from build123d import *

# Parameters (mm, degrees)
EXTRUDE_1_DEPTH      = 5
EXTRUDE_1_DEPTH_BACK = 2
SKETCH_2_W           = 30
SKETCH_2_H           = 5
EXTRUDE_2_DEPTH      = 25
SKETCH_3_W           = 60
SKETCH_3_H           = 10
EXTRUDE_3_DEPTH      = 25


with BuildPart() as part:
    # 草圖1 → 填料-伸長1 (new, two sides: drawn at the far end of the back side and taken through both)
    with BuildSketch(Plane(origin=(0, 0, 0), x_dir=(1, 0, 0), z_dir=(0, 1, 0)).offset(-EXTRUDE_1_DEPTH_BACK)):
        Polygon((-60, 65), (-60, 40), (-30, 40), (-30, 65), (30, 65), (30, 40), (60, 40), (60, 65), (100, 65), (100, -65), (60, -65), (60, -40), (30, -40), (30, -65), (-30, -65), (-30, -40), (-60, -40), (-60, -65), (-100, -65), (-100, 65), align=None)
    extrude(amount=EXTRUDE_1_DEPTH + EXTRUDE_1_DEPTH_BACK)

    # 草圖2 → 填料-伸長2 (add)
    with BuildSketch(Plane(origin=(0, 5, 0), x_dir=(1, 0, 0), z_dir=(0, 1, 0))):
        with Locations((-45, 37.5)):
            Rectangle(SKETCH_2_W, SKETCH_2_H)
        with Locations((-45, -37.5)):
            Rectangle(SKETCH_2_W, SKETCH_2_H)
        with Locations((45, -37.5)):
            Rectangle(SKETCH_2_W, SKETCH_2_H)
        with Locations((45, 37.5)):
            Rectangle(SKETCH_2_W, SKETCH_2_H)
    extrude(amount=EXTRUDE_2_DEPTH)

    # 草圖3 → 填料-伸長3 (add)
    with BuildSketch(Plane(origin=(0, 5, 0), x_dir=(1, 0, 0), z_dir=(0, 1, 0))):
        Polygon((70, -65), (100, -65), (100, 65), (70, 65), (70, 55), (90, 55), (90, -55), (70, -55), align=None)
        with Locations((0, 60)):
            Rectangle(SKETCH_3_W, SKETCH_3_H)
        with Locations((0, -60)):
            Rectangle(SKETCH_3_W, SKETCH_3_H)
        Polygon((-100, 65), (-100, -65), (-70, -65), (-70, -55), (-90, -55), (-90, 55), (-70, 55), (-70, 65), align=None)
    extrude(amount=EXTRUDE_3_DEPTH)


solid = part.part
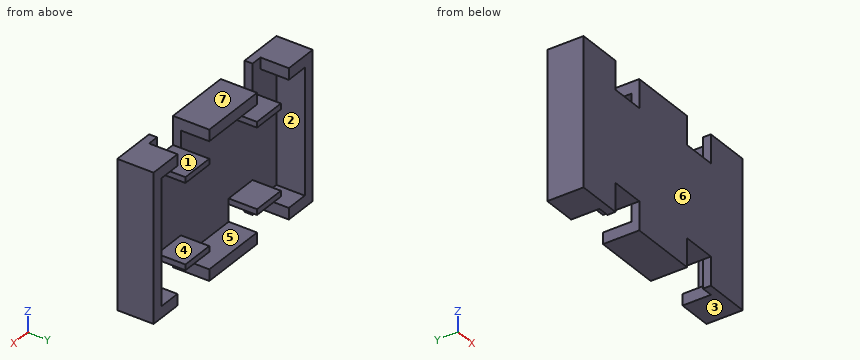
The model under review builds one solid part; all positions refer to its coordinate system, in mm. Face numbers are marked on the shaded views. A direction names the side the tool comes from. Give positions to 0.01 mm unless a question says otherwise; leave off trailing zeros. Order: outer loops, then holes, each group sorted by start corner. A loop starts at its lowest first (then second) coordinate and runs counter-clockwise, first axis right, second up. Notation, with made-up numbers: M 66,74 L 111,74 A19 cw 111,94 Z; hole C 86,62 d8. An arc over 180 degrees is marked long. Answer in a Markdown table with one row per item. Add a question column.
1. Mouldability with a two-part tool opening along Z and no side actions: class the marked faces 4, 5, 6 and 7 as released by +Z, released by -Z, zero draft, split by the parting line, or undercut.
2. Add section A-A on z = 48.5. State the section outline as (x, y) points, plus the area to 3 significant figures.
3. Machinability: for the marked faces 1, 2 and 3, which of the approach directions +Z, -Z, +X, -X, +Y, -Y give a long, thin tool a straight path to every point of the face, cutting with its end or side? Answer none if there is none.
4. Add section C-C on x = 37.5. State the section outline as (y, z) points, plus the area to 3 significant figures.
5. For pin 1 Ø9 at (x, y) = (43.5, 7) entering from -Z, flat-tipped, find the tip position at first contact; note if it passes through.
6. To check wall thickness, follow line 1 along X through (y, z) = (1.5, -57); line 2 along X through (y, z) = (10.5, 55.5); line 3 along X through (y, z) = (27.5, -43.5). State the ranges of each line that lie inside material, in increasing order.
7. Add section D-D on z = 13.5. State the section outline as (x, y) points, plus the area to 3 significant figures.
8. Add section B-B on y = 3. State the section outline as (x, z) points.
The answers:
| question | item | result |
|---|---|---|
| 1 | face 4 | undercut |
| 1 | face 5 | undercut |
| 1 | face 6 | zero draft |
| 1 | face 7 | released by +Z |
| 2 | outline | M -100,-2 L -60,-2 L -60,5 L -90,5 L -90,30 L -100,30 Z; M -30,-2 L 30,-2 L 30,5 L -30,5 Z; M 60,-2 L 100,-2 L 100,30 L 90,30 L 90,5 L 60,5 Z |
| 2 | area | 1,480 mm2 |
| 3 | face 1 | +Z, +Y, -Y |
| 3 | face 2 | +Y |
| 3 | face 3 | -Z, +X, -X, +Y, -Y |
| 4 | outline | M -2,-40 L 30,-40 L 30,-35 L 5,-35 L 5,35 L 30,35 L 30,40 L -2,40 Z |
| 4 | area | 810 mm2 |
| 5 | pin 1 | z = -40 |
| 6 | line 1 | -100 to -60, -30 to 30, 60 to 100 |
| 6 | line 2 | -100 to -70, -30 to 30, 70 to 100 |
| 6 | line 3 | -100 to -90, 90 to 100 |
| 7 | outline | M -100,-2 L 100,-2 L 100,30 L 90,30 L 90,5 L -90,5 L -90,30 L -100,30 Z |
| 7 | area | 1,900 mm2 |
| 8 | outline | M -100,-65 L -60,-65 L -60,-40 L -30,-40 L -30,-65 L 30,-65 L 30,-40 L 60,-40 L 60,-65 L 100,-65 L 100,65 L 60,65 L 60,40 L 30,40 L 30,65 L -30,65 L -30,40 L -60,40 L -60,65 L -100,65 Z |
